Autodesk Inventor part; units mm, degrees
ref_plane "YZ Plane" through (0, 0, 0) normal (1, 0, 0) x (0, 1, 0)
ref_plane "XZ Plane" through (0, 0, 0) normal (0, 1, 0) x (-1, 0, 0)
ref_plane "XY Plane" through (0, 0, 0) normal (0, 0, 1) x (1, 0, 0)
sketch "Boceto1" plane through (0, 0, 0) normal (0, 1, 0) x (-1, 0, 0)
  line L0 (0, 0) -> (51, 0)
  line L1 (51, 0) -> (51, -28)
  line L2 (51, -28) -> (0, -28)
  line L3 (0, -28) -> (0, 0)
  line L4 (51, 0) -> (51, -18.5)
  line L5 (51, -18.5) -> (42, -18.5)
  circle A0 centre (42, -18.5) radius 1.5
  line L6 (0, 0) -> (0, -14.5)
  line L7 (0, -14.5) -> (4.25, -14.5)
  circle A1 centre (4.25, -14.5) radius 1.5
  line L8 (51, 0) -> (51, -14)
  line L9 (51, -14) -> (55, -14)
  line L10 (55, -14) -> (55, -9)
  line L11 (55, -9) -> (51, -9)
  line L12 (55, -14) -> (55, -19)
  line L13 (55, -19) -> (51, -19)
  dimension "d0" = 51
  dimension "d1" = 28
  dimension "d2" = 18.5
  dimension "d3" = 9
  dimension "d4" = 3
  dimension "d5" = 14.5
  dimension "d6" = 4.25
  dimension "d7" = 3
  dimension "d8" = 14
  dimension "d9" = 4
  dimension "d10" = 5
  dimension "d11" = 5
extrude "Extrusión1" add sketch "Boceto1" along normal blind 2
properties part number "arm_2_microservo_case"
Here's how the part is built. I have some questions about the finished solid (model axes, mm). A direction names the side the tool comes from. Coordinates: 2 decimals unless noted, no trailing zeros. Order: outer loops, then holes, each group sorted by start corner. A loop starts at its lowest first (then second) coordinate and runs counter-clockwise, first axis right, second up. Notation, with made-up numbers: M -15,17.5 L 9,17.5 A25 cw 9,40.5 Z; hole C -9,17 d4. An arc over 180 degrees is marked long. Answer as CSV lines item,"result".
Item 1: If I drill on line 1 (Z direction, x = -42, y = 1.2); line 2 (Z direction, x = -4.25, y = 1.3); line 3 (X direction, y = 1, z = -14.5), over which ranges is the centre line in solid material (lowest first)?
Results found:
line 1,"-28 to -20, -17 to 0"
line 2,"-28 to -16, -13 to 0"
line 3,"-55 to -5.75, -2.75 to 0"
Item 2: We'd pull the mould along Z, two halves only. Please class faces 4 (the face through (-40.89, 0.99, -19.51)), 5 (the face through (-27, 2, -14)), 6 (the face through (-53, 1, -9)), 7 (the face through (-5.636, 0.986, -13.925)): +Z half, -Z half, draft (parallel to the pull), parting line (faces both ways), or undercut.
Results found:
face 4,"undercut"
face 5,"draft"
face 6,"+Z half"
face 7,"undercut"
Item 3: On a 3-axis mill with a long thin cutter (end or side, diameter ignored), from which of +Z, -Z, +X, -X, +Y, -Y can I reach the whole of each face in a straight line? I mean faces 1 (the face through (-25, 1, 0)), 2 (the face through (-53, 1, -19)), 3 (the face through (-51, 1, -4)). Say none if no direction works.
Results found:
face 1,"+Z, +X, -X, +Y, -Y"
face 2,"-Z, -X, +Y, -Y"
face 3,"+Z, -X, +Y, -Y"
Item 4: Imagine slicing it at A-A on z = -14.5. Write out the boundary of the cut face in (x, y).
Results found:
outline,"M -55,0 L -5.75,0 L -5.75,2 L -55,2 Z; M -2.75,0 L 0,0 L 0,2 L -2.75,2 Z"
Item 5: Imagine slicing it at B-B on x = -42. Write out the boundary of the cut face in (y, z).
Results found:
outline,"M 0,-28 L 2,-28 L 2,-20 L 0,-20 Z; M 0,-17 L 2,-17 L 2,0 L 0,0 Z"
Item 6: For pin 1 (2.5 mm diameter, centred on x = -42, z = -18.5, fed in from +Y); pin 2 (0.6 mm diameter, centred on x = -52.5, y = 1, fed in from +Z); pin 3 (1 mm diameter, centred on x = -52.5, y = 1.5, fed in from -Z); pin 4 (1 mm diameter, centred on y = 0.5, z = -5.5, fed in from -X), each with a flat end and sliding along its axis, tell me the tip position at first contact or that it passes through.
Results found:
pin 1,"through"
pin 2,"z = -9"
pin 3,"z = -19"
pin 4,"x = -51"
Item 7: Imagine slicing it at C-C on y = 0.35. Write out the boundary of the cut face in (x, z), plus the area to 3 significant figures.
Results found:
outline,"M -55,-19 L -51,-19 L -51,-28 L 0,-28 L 0,0 L -51,0 L -51,-9 L -55,-9 Z; hole C -42,-18.5 d3; hole C -4.25,-14.5 d3"
area,"1,450 mm2"
Item 8: Imagine slicing it at D-D on z = -6. Write out the boundary of the cut face in (x, y).
Results found:
outline,"M -51,0 L 0,0 L 0,2 L -51,2 Z"
